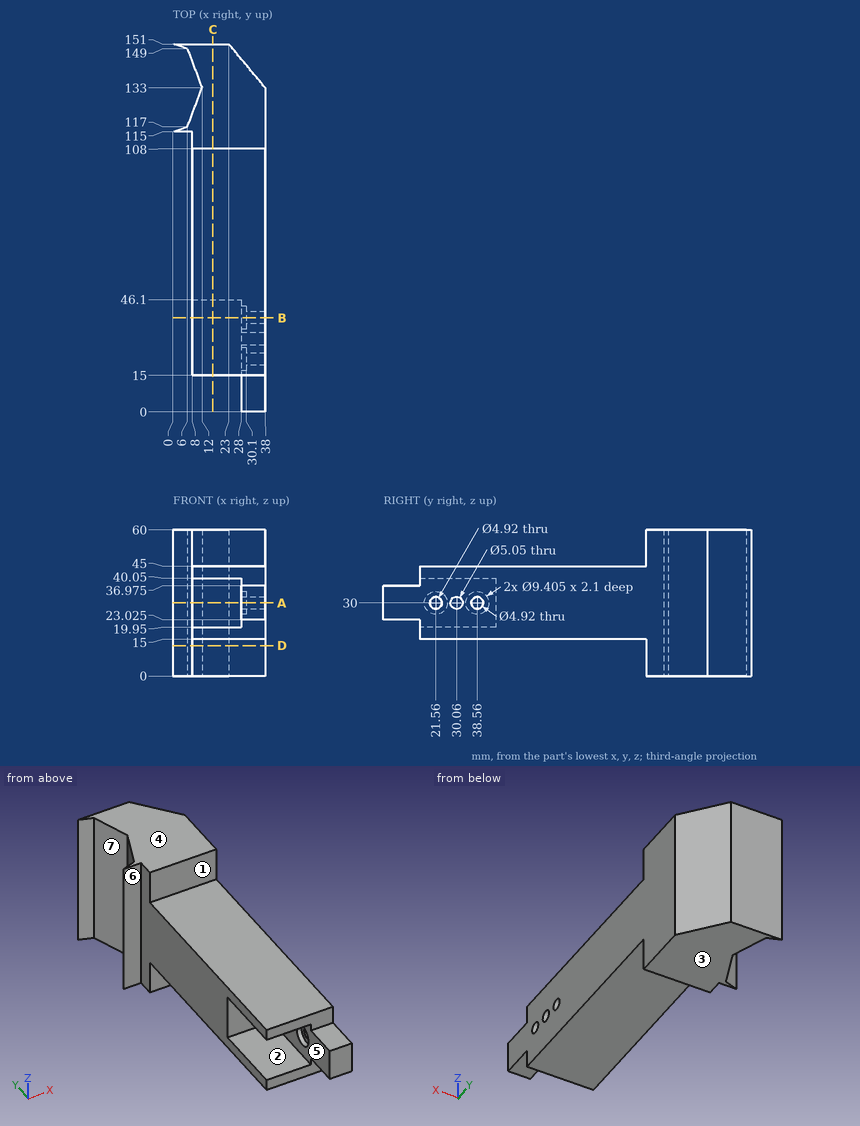
Drawing for the job (mm, zero at the part's lowest x, y, z). A direction names the side the tool comes from. Round coordinates to 2 decimals unless told otherwise and drop trailing zeros. Write each loop counter-clockwise with the first axis right and the second up, starting at its lowest first coordinate (ties: lowest second). Pieces come first, ordered by that corner, then holes. Notation, with made-up numbers: M 54.25,-28 L 71.25,-28 A21 cw 71.25,-5 Z; hole C -25.75,-2 d4. An arc over 180 degrees is marked long. Answer as a JSON object with one key per item and string values. Group by question number.
(1) Which spindle directions (+Z, -Z, +X, -X, +Y, -Y) get a long thin tool onto all of the face, cutting with end or side? Do the marked faces 5, 6 and 7. Say none if no direction does.
(2) Cut at C-C (x = 16.5). Give the cut face in (y, z), and give its area (3 significant figures).
(3) Cut at B-B (y = 38.56). Give the cut face in (x, z).
(4) Flat gauge pins, fed straight in: pin 1 (6 mm diameter, centred on x = 17, y = 31.5, fed in from -Z); pin 2 (3 mm diameter, centred on x = 35, y = 6.5, fed in from +Z) (3 decimals); pin 3 (2.5 mm diameter, centred on x = 18, z = 42.5, fed in from -Y); pin 4 (8 mm diameter, centred on y = 21.56, z = 30, fed in from +X). Where does each tip first touch, or does it go through?
(5) Cut at A-A (z = 30). Give the number of separate pieces and of enclosed holes in the cut face, and give its area (3 significant figures).
(6) Drill centre lines: L1, parallel to Z at x = 31, y = 30; L2, parallel to Z at x = 21, y = 18; L3, parallel to Y at x = 19.5, z = 46.5. Where is each one in solid material? Low to high.
(7) Cut at D-D (z = 12.5). Give the cut face in (x, y), and give its area (3 significant figures).
(8) Mould opens along Z. For the marked faces 1, 2, 3 and 4 say: pulls with the +Z half, pulls with the -Z half, needs draft (parallel to the pull), parting line crosses it, or undercut.
Responses:
{
 "1": {"face 5": "-X, -Y", "face 6": "+Z, -Z, -X, -Y", "face 7": "+Z, -Z, -X"},
 "2": {"outline": "M 15,15 L 108,15 L 108,0 L 151,0 L 151,60 L 108,60 L 108,45 L 15,45 L 15,40.05 L 46.1,40.05 L 46.1,19.95 L 15,19.95 Z", "area": "4,740 mm2"},
 "3": {"outline": "M 8,15 L 38,15 L 38,27.54 L 30.1,27.54 L 30.1,25.3 L 28,25.3 L 28,19.95 L 8,19.95 Z; M 8,40.05 L 28,40.05 L 28,34.7 L 30.1,34.7 L 30.1,32.46 L 38,32.46 L 38,45 L 8,45 Z"},
 "4": {"pin 1": "stops at z = 15", "pin 2": "stops at z = 36.975", "pin 3": "stops at y = 15", "pin 4": "stops at x = 38"},
 "5": {"separate pieces": "4", "enclosed holes": "0", "area": "3,290 mm2"},
 "6": {"L1": "z = 15 to 27.48, 32.52 to 45", "L2": "z = 15 to 19.95, 40.05 to 45", "L3": "y = 108 to 151"},
 "7": {"outline": "M 0,115 L 8,115 L 8,108 L 38,108 L 38,133 L 23,151 L 0,151 L 6,149 L 12,133 L 6,117 Z", "area": "1,140 mm2"},
 "8": {"face 1": "needs draft", "face 2": "undercut", "face 3": "pulls with the -Z half", "face 4": "pulls with the +Z half"}
}
